Here's how the part is built. I have some questions about the finished solid (model axes, mm). Round coordinates to 2 decimals unless told otherwise and drop trailing zeros. Write each loop counter-clockwise with the first axis right and the second up, starting at its lowest first coordinate (ties: lowest second). Pieces come first, ordered by that corner, then holes. Notation, with made-up numbers: (-4, 37) -> (42, 37) arc R18 cw to (42, 54) -> close; hole circle Ø10 at (-35.5, 38). An arc over 180 degrees is marked (long way). Answer in a Markdown table with one row per item.
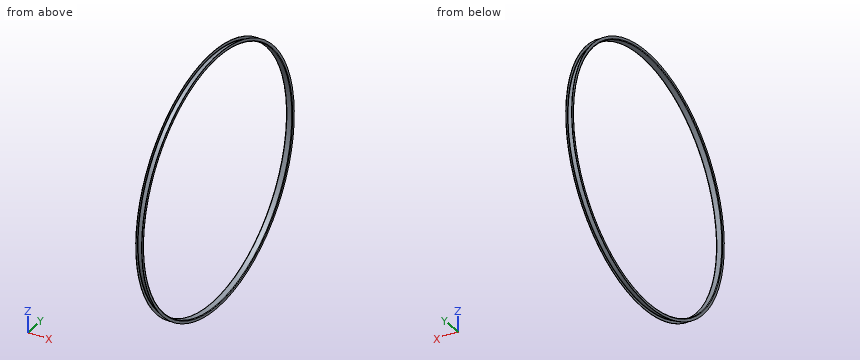
from build123d import *


with BuildPart() as part:
    # Sketch1 → Revolve1 (revolve)
    with BuildSketch(Plane.XY, mode=Mode.PRIVATE) as revolve1_sk:
        with BuildLine():
            Line((-38, 75.537190083), (-38, 59.537190083))
            ThreePointArc((-38, 59.537190083), (-36.828427125, 56.708762958), (-34, 55.537190083))
            Line((-34, 55.537190083), (-2, 55.537190083))
            ThreePointArc((-2, 55.537190083), (0.828427125, 56.708762958), (2, 59.537190083))
            Line((2, 59.537190083), (2, 75.537190083))
            Line((2, 75.537190083), (0, 75.537190083))
            Line((0, 75.537190083), (0, 59.537190083))
            ThreePointArc((0, 59.537190083), (-0.585786438, 58.12297652), (-2, 57.537190083))
            Line((-2, 57.537190083), (-34, 57.537190083))
            ThreePointArc((-34, 57.537190083), (-35.414213562, 58.12297652), (-36, 59.537190083))
            Line((-36, 59.537190083), (-36, 75.537190083))
            Line((-36, 75.537190083), (-38, 75.537190083))
        make_face()
    revolve(revolve1_sk.sketch.rotate(Axis((63.944474241, -749.462809917, 0), (-1, 0, 0)), 90), axis=Axis((63.944474241, -749.462809917, 0), (-1, 0, 0)))


solid = part.part
1) For pin 1 (3 mm diameter, centred on x = -24, y = -1387.5, fed in from +Z); pin 2 (5 mm diameter, centred on x = -23.5, z = -600, fed in from +Y); pin 3 (3 mm diameter, centred on x = -3.5, y = -258, fed in from +Z), each with a flat end and sliding along its axis, tell me the tip position at first contact or that it passes through.
Response:
| item | result |
|---|---|
| pin 1 | stops at z = 496.05 |
| pin 2 | stops at y = -207.02 |
| pin 3 | stops at z = 641.24 |
2) I want a section at A-A, the plane z = 0. List the corners of the cut face in (x, y) for me.
Response:
| item | result |
|---|---|
| outline | (-38, -1574.46) -> (-36, -1574.46) -> (-36, -1558.46) arc R2 cw to (-34, -1556.46) -> (-2, -1556.46) arc R2 cw to (0, -1558.46) -> (0, -1574.46) -> (2, -1574.46) -> (2, -1558.46) arc R4 ccw to (-2, -1554.46) -> (-34, -1554.46) arc R4 ccw to (-38, -1558.46) -> close; (-38, 59.54) arc R4 ccw to (-34, 55.54) -> (-2, 55.54) arc R4 ccw to (2, 59.54) -> (2, 75.54) -> (0, 75.54) -> (0, 59.54) arc R2 cw to (-2, 57.54) -> (-34, 57.54) arc R2 cw to (-36, 59.54) -> (-36, 75.54) -> (-38, 75.54) -> close |
3) I want a section at B-B, the plane x = -27. List the corners of the cut face in (y, z) for me, and give its area (3 significant figures).
Response:
| item | result |
|---|---|
| outline | circle Ø1614 at (-749.46, 0); hole circle Ø1610 at (-749.46, 0) |
| area | 10,100 mm^2 |
4) I need wall thicknesses on line 1 (X direction, y = -1190.5, z = 677); line 2 (Y direction, x = -20, z = 14); line 3 (Y direction, x = -20, z = 0). Which ranges of each line are inside material? Lowest first, please. Write a range as [from, to].
Response:
| item | result |
|---|---|
| line 1 | x = [-37.87, -35.72], [-0.28, 1.87] |
| line 2 | y = [-1556.34, -1554.34], [55.42, 57.42] |
| line 3 | y = [-1556.46, -1554.46], [55.54, 57.54] |
